from build123d import *

# Parameters (mm, degrees)
SKETCH1_R           = 19.9
BOSS_EXTRUDE1_DEPTH = 7
SKETCH2_R           = 22
BOSS_EXTRUDE2_DEPTH = 1
SKETCH3_R           = 1.5
SKETCH3_R_2         = 1.6
CUT_EXTRUDE1_DEPTH  = 9
SKETCH4_R           = 3.25
CUT_EXTRUDE2_DEPTH  = 4
CHAMFER1_SIZE       = 1


with BuildPart() as part:
    # Sketch1 → Boss-Extrude1 (new body)
    with BuildSketch(Plane(origin=(0, 0, 0), x_dir=(1, 0, 0), z_dir=(0, 1, 0))):
        Circle(SKETCH1_R)
    extrude(amount=BOSS_EXTRUDE1_DEPTH)

    # Sketch2 → Boss-Extrude2 (add)
    with BuildSketch(Plane(origin=(0, 7, 0), x_dir=(1, 0, 0), z_dir=(0, 1, 0))):
        Circle(SKETCH2_R)
    extrude(amount=BOSS_EXTRUDE2_DEPTH)

    # Sketch3 → Cut-Extrude1 (cut, through all)
    with BuildSketch(Plane(origin=(0, 8, 0), x_dir=(1, 0, 0), z_dir=(0, 1, 0))):
        with Locations((0, 16)):
            Circle(SKETCH3_R)
        with Locations((13.856406461, 8)):
            Circle(SKETCH3_R)
        with Locations((13.856406461, -8)):
            Circle(SKETCH3_R)
        with Locations((0, -16)):
            Circle(SKETCH3_R)
        with Locations((-13.856406461, -8)):
            Circle(SKETCH3_R)
        with Locations((-13.856406461, 8)):
            Circle(SKETCH3_R)
        with Locations((-8, 13.856406461)):
            Circle(SKETCH3_R_2)
        with Locations((-16, 0)):
            Circle(SKETCH3_R_2)
        with Locations((-8, -13.856406461)):
            Circle(SKETCH3_R_2)
        with Locations((8, -13.856406461)):
            Circle(SKETCH3_R_2)
        with Locations((16, 0)):
            Circle(SKETCH3_R_2)
        with Locations((8, 13.856406461)):
            Circle(SKETCH3_R_2)
    extrude(amount=-CUT_EXTRUDE1_DEPTH, mode=Mode.SUBTRACT)

    # Sketch4 → Cut-Extrude2 (cut)
    with BuildSketch(Plane(origin=(0, 8, 0), x_dir=(1, 0, 0), z_dir=(0, 1, 0))):
        with Locations((-8, 13.856406461)):
            Circle(SKETCH4_R)
        with Locations((8, 13.856406461)):
            Circle(SKETCH4_R)
        with Locations((16, 0)):
            Circle(SKETCH4_R)
        with Locations((8, -13.856406461)):
            Circle(SKETCH4_R)
        with Locations((-8, -13.856406461)):
            Circle(SKETCH4_R)
        with Locations((-16, 0)):
            Circle(SKETCH4_R)
    extrude(amount=-CUT_EXTRUDE2_DEPTH, mode=Mode.SUBTRACT)

    # Chamfer1
    chamfer1_edges = [part.edges().sort_by_distance(p)[0] for p in [
        (-19.9, 0, 0),
    ]]
    chamfer(chamfer1_edges, length=CHAMFER1_SIZE)


solid = part.part
Work out the finished part from the listing and answer in its coordinate system (mm). A direction names the side the tool comes from. Round coordinates to 2 decimals unless told otherwise and drop trailing zeros. Loops run counter-clockwise (first coordinate to the right, second up) from the corner with the lowest first, then second, coordinate; pieces in that order, holes last. Notation, with made-up numbers: (-7, 8.25) - (-3, 8.25) arc R23 ccw to (-3, 44.25) - close; hole circle Ø10 at (50.25, 39). An arc over 180 degrees is marked (long way). One line per item, written item: value.
Q1. Find section A-A on x = 0. Give the vertices of the cut face in (y, z).
Check values:
outline: (0, -18.9) - (1, -19.9) - (7, -19.9) - (7, -22) - (8, -22) - (8, -17.5) - (0, -17.5) - close; (0, -14.5) - (8, -14.5) - (8, 14.5) - (0, 14.5) - close; (0, 17.5) - (8, 17.5) - (8, 22) - (7, 22) - (7, 19.9) - (1, 19.9) - (0, 18.9) - close
Q2. Find section B-B on y = 2. State how many separate pieces and enclosed holes the cut face has, and give its area (3 significant figures).
Check values:
separate pieces: 1
enclosed holes: 12
area: 1,150 mm2
Q3. For faces 1 (the cylindrical face through (-1.11, 4.06, -17.01)), 2 (the flat face through (17.4, 4, 1.4)), determine the directions among +Z, -Z, +X, -X, +Y, -Y from which every point of the face is accessible in a straight line to the end or side of a thin tool.
Check values:
face 1: +Y, -Y
face 2: +Y
Q4. The mould has two halves that part along X. Classify faces 3 (the flat face through (-5, 7, 19.5)), 4 (the cylindrical face through (-0.325, 4.056, 17.464)): +X half, -X half, draft (parallel to the pull), parting line (faces both ways), or undercut.
Check values:
face 3: draft
face 4: undercut
Q5. Each of these flat-tipped pins is pushed along its axis until it touches: pin 1 Ø3 at (x, z) = (8, 13.86) entering from -Y; pin 2 Ø3 at (y, z) = (2.5, 6.5) entering from -X; pin 3 Ø3 at (x, z) = (8, -14) entering from +Y; pin 4 Ø2 at (x, y) = (-15.5, 3.5) entering from +Z. Where does it stop, or does it pass through?
Check values:
pin 1: through
pin 2: x = -19.26
pin 3: y = 4
pin 4: z = 13.63
Q6. Straight lines are drawn through the part: probe 1 along X at (y, z) = (6.6, 0); probe 2 along Z at (x, y) = (-8, 6.8); probe 3 along X at (y, z) = (6.25, 12.5). For each, find the intervals that lie inside material, in ascending order.
Check values:
probe 1: -19.9 to -19.25, -12.75 to 12.75, 19.25 to 19.9
probe 2: -18.22 to -17.11, -10.61 to 10.61, 17.11 to 18.22
probe 3: -15.48 to -10.95, -5.05 to 5.05, 10.95 to 15.48
